```python
from build123d import *

# Parameters (mm, degrees)
F0_W     = 840
F0_H     = 1840
F1_DEPTH = 1800
F2_T     = 25.4


with BuildPart() as f1:
    # F0 (on Top) → F1 (new body)
    with BuildSketch(Plane.XY):
        Rectangle(F0_W, F0_H)
    extrude(amount=-F1_DEPTH)

    # F2
    f2_openings = [f1.faces().sort_by_distance(p)[0] for p in [
        (420, 0, -900),
    ]]
    offset(amount=F2_T, openings=f2_openings, kind=Kind.INTERSECTION)


solid = f1.part
```
The listing builds one solid part. Answer for the finished solid, in the listing's coordinates (mm). A direction names the side the tool comes from. Coordinates: 2 decimals unless noted, no trailing zeros. Write each loop counter-clockwise with the first axis right and the second up, starting at its lowest first coordinate (ties: lowest second). Pieces come first, ordered by that corner, then holes. Notation, with made-up numbers: (44, 10) - (80, 10) arc R7 cw to (80, 16) - close; hole circle Ø6 at (-19.75, -26). An arc over 180 degrees is marked (long way). Return JSON: item names as keys, results as strings. Group by question number.
1. Given pin 1 (2 mm diameter, centred on y = -569, z = -352, fed in from +X), flat-ended and moving along its own axis, determine where the tip first touches the part or whether it passes through.
2. A cutting plane is placed at B-B, the plane z = -1384. Determine the outline of the cut face in (x, y).
3. Which of the six approach directions +Z, -Z, +X, -X, +Y, -Y give full straight-line access (tool end or side, diameter ignored) to faces 1 (the flat face through (-6, 13, -1800)), 2 (the flat face through (-19, 945.4, -887))?
4. Straight lines are drawn through the part: L1, parallel to Y at x = 266, z = -1363; L2, parallel to Z at x = -283.5, y = -368; L3, parallel to X at y = -428, z = -441.5. For each, find the intervals that lie inside material, in ascending order.
5. A cutting plane is placed at A-A, the plane x = -198.5. Determine the outline of the cut face in (y, z).
6. A cutting plane is placed at C-C, the plane y = 7.5. Determine the outline of the cut face in (x, z).
7. Determine the mould class of faces 3 (the flat face through (-19, 13, -1825.4)), 4 (the flat face through (-6, 920, -887)), 5 (the flat face through (-445.4, -13, -887)), 6 (the flat face through (-19, 13, 25.4)) for opening direction Z: released by +Z, released by -Z, zero draft, split by the parting line, or undercut.
Ans:
{
 "1": {"pin 1": "x = -420"},
 "2": {"outline": "(-445.4, -945.4) - (420, -945.4) - (420, -920) - (-420, -920) - (-420, 920) - (420, 920) - (420, 945.4) - (-445.4, 945.4) - close"},
 "3": {"face 1": "+X", "face 2": "+Z, -Z, +X, -X, +Y"},
 "4": {"L1": "-945.4 to -920, 920 to 945.4", "L2": "-1825.4 to -1800, 0 to 25.4", "L3": "-445.4 to -420"},
 "5": {"outline": "(-945.4, -1825.4) - (945.4, -1825.4) - (945.4, 25.4) - (-945.4, 25.4) - close; hole (-920, -1800) - (920, -1800) - (920, 0) - (-920, 0) - close"},
 "6": {"outline": "(-445.4, -1825.4) - (420, -1825.4) - (420, -1800) - (-420, -1800) - (-420, 0) - (420, 0) - (420, 25.4) - (-445.4, 25.4) - close"},
 "7": {"face 3": "released by -Z", "face 4": "undercut", "face 5": "zero draft", "face 6": "released by +Z"}
}
